The listing builds one solid part. Answer for the finished solid, in the listing's coordinates (mm). A direction names the side the tool comes from. Coordinates: 2 decimals unless noted, no trailing zeros. Write each loop counter-clockwise with the first axis right and the second up, starting at its lowest first coordinate (ties: lowest second). Pieces come first, ordered by that corner, then holes.
from build123d import *

# Parameters (mm, degrees)
F0_W     = 24
F0_H     = 18
F0_R     = 2.5
F0_W_2   = 8
F0_H_2   = 3
F1_DEPTH = 0.8
F2_D     = 2.8
F3_DEPTH = 2
F4_SIZE2 = 1.99999
F4_SIZE  = 0.99999
F5_SIZE2 = 0.99999
F5_SIZE  = 1.99999
F6_DEPTH = 6.8
F7_DEPTH = 9.8
F8_SIZE2 = 8.99999
F8_SIZE  = 0.99999


# Not quite as in the source:
# - a fillet or chamfer is up to 0.001 mm smaller than in the source, because OpenCascade refuses the exact size


with BuildPart() as f1:
    # F0 (on Front) → F1 (new body)
    with BuildSketch(Plane.XZ):
        Rectangle(F0_W, F0_H)
        with Locations((-2, -6)):
            Circle(F0_R, mode=Mode.SUBTRACT)
        with Locations((-2.5, 6)):
            Rectangle(F0_W_2, F0_H_2, mode=Mode.SUBTRACT)
        with Locations((-2.5, 6)):
            Rectangle(F0_W_2, F0_H_2)
        with Locations((-2, -6)):
            Circle(F0_R)
    extrude(amount=F1_DEPTH)

    # F2 (through all)
    with Locations(Plane(origin=(0, 0, 0), x_dir=(1, 0, 0), z_dir=(0, 1, 0))):
        with Locations((-9.3, -6), (9.11, -6)):
            Hole(F2_D / 2)

    # F0 (on Front) → F3 (join)
    with BuildSketch(Plane.XZ):
        with Locations((-2.5, 6)):
            Rectangle(F0_W_2, F0_H_2)
        with Locations((-2, -6)):
            Circle(F0_R)
    extrude(amount=-F3_DEPTH)

    # F4 (size 1 and 2 in the source; OpenCascade refuses exactly that, so slightly less here)
    f4_edges = [f1.edges().sort_by_distance(p)[0] for p in [
        (-2.5, 2, 4.5),
        (-2.5, 2, 7.5),
    ]]
    f4_side = f1.faces().sort_by_distance((-2.5, 2, 6))[0]
    chamfer(f4_edges, length=F4_SIZE, length2=F4_SIZE2, reference=f4_side)

    # F5 (size 2 and 1 in the source; OpenCascade refuses exactly that, so slightly less here)
    f5_edges = [f1.edges().sort_by_distance(p)[0] for p in [
        (-4.5, 2, -6),
    ]]
    f5_side = f1.faces().sort_by_distance((-4.5, 1, -6))[0]
    chamfer(f5_edges, length=F5_SIZE, length2=F5_SIZE2, reference=f5_side)

    # F0 (on Front) → F6 (join)
    with BuildSketch(Plane.XZ):
        with Locations((-2, -6)):
            Circle(F0_R)
    extrude(amount=F6_DEPTH)

    # F0 (on Front) → F7 (join)
    with BuildSketch(Plane.XZ):
        with Locations((-2.5, 6)):
            Rectangle(F0_W_2, F0_H_2)
    extrude(amount=F7_DEPTH)

    # F8 (size 1 and 9 in the source; OpenCascade refuses exactly that, so slightly less here)
    f8_edges = [f1.edges().sort_by_distance(p)[0] for p in [
        (-2.5, -9.8, 7.5),
        (-2.5, -9.8, 4.5),
    ]]
    f8_side = f1.faces().sort_by_distance((-2.5, -9.8, 6))[0]
    chamfer(f8_edges, length=F8_SIZE, length2=F8_SIZE2, reference=f8_side)


solid = f1.part
Q1. Given pin 1 (1 mm diameter, centred on x = -7.5, z = -7, fed in from -Y); pin 2 (2.5 mm diameter, centred on x = -2.5, z = -5.5, fed in from -Y); pin 3 (0.6 mm diameter, centred on y = 1, z = 6, fed in from -X), each flat-ended and moving along its own axis, determine where each tip first touches the part or whether it passes through.
Answers below:
pin 1: stops at y = -0.8
pin 2: stops at y = -6.8
pin 3: stops at x = -6.5
Q2. The part is cut by section A-A, the plane x = -9.3. Write down the section's boundary in (y, z).
Answers below:
outline: (-0.8, -9) - (0, -9) - (0, 4.6) - (-0.8, 4.6) - close; (-0.8, 7.4) - (0, 7.4) - (0, 9) - (-0.8, 9) - close
Q3. Determine the mould class of faces 4 (the face through (-2.556, -5.237, 4.993)), 5 (the face through (-3, 1, 7)), 6 (the face through (-6.5, 1, 6)) for opening direction Z: released by +Z, released by -Z, zero draft, split by the parting line, or undercut.
Answers below:
face 4: undercut
face 5: released by +Z
face 6: zero draft
Q4. Find the intervals of material crossed by probe 1 along X at (y, z) = (-0.25, 6); probe 2 along Z at (x, y) = (-9.3, -0.45); probe 3 along Y at (x, z) = (1.25, -2.75), in increasing order.
Answers below:
probe 1: x = -12 to -10.7, -7.9 to 7.71, 10.51 to 12
probe 2: z = -9 to 4.6, 7.4 to 9
probe 3: y = -0.8 to 0
Q5. The part is cut by section B-B, the plane z = 6. Write down the section's boundary in (x, y).
Answers below:
outline: (-12, -0.8) - (-10.7, -0.8) - (-10.7, 0) - (-12, 0) - close; (-7.9, -0.8) - (-6.5, -0.8) - (-6.5, -9.8) - (1.5, -9.8) - (1.5, -0.8) - (7.71, -0.8) - (7.71, 0) - (1.5, 0) - (1.5, 2) - (-6.5, 2) - (-6.5, 0) - (-7.9, 0) - close; (10.51, -0.8) - (12, -0.8) - (12, 0) - (10.51, 0) - close
Q6. Which of the six approach directions +Z, -Z, +X, -X, +Y, -Y give full straight-line access (tool end or side, diameter ignored) to faces 1 (the face through (-6.5, -4, 6)), 2 (the face through (-3.84, -3.76, -4.31)), 3 (the face through (0, 0, 0))?
Answers below:
face 1: +Z, -Z, -X, -Y
face 2: -Y
face 3: +Y
Q7. The part is cut by section D-D, the plane y = -4.5. Write down the section's boundary in (x, z).
Answers below:
outline: (-6.5, 4.91) - (1.5, 4.91) - (1.5, 7.09) - (-6.5, 7.09) - close; circle Ø5 at (-2, -6)
